```python
from build123d import *

# Parameters (mm, degrees)
SKETCH1_W           = 450
SKETCH1_H           = 25.4
BOSS_EXTRUDE1_DEPTH = 25.4
SKETCH2_W           = 23
SKETCH2_H           = 23
CUT_EXTRUDE1_DEPTH  = 450
CUT_EXTRUDE2_DEPTH  = 25.4


with BuildPart() as part:
    # Sketch1 → Boss-Extrude1 (new body)
    with BuildSketch(Plane(origin=(0, 0, 0), x_dir=(1, 0, 0), z_dir=(0, 1, 0))):
        with Locations((225, 12.7)):
            Rectangle(SKETCH1_W, SKETCH1_H)
    extrude(amount=BOSS_EXTRUDE1_DEPTH)

    # Sketch2 → Cut-Extrude1 (cut)
    with BuildSketch(Plane(origin=(450, 0, 0), x_dir=(0, 0, -1), z_dir=(1, 0, 0))):
        with Locations((12.7, 12.7)):
            Rectangle(SKETCH2_W, SKETCH2_H)
    extrude(amount=-CUT_EXTRUDE1_DEPTH, mode=Mode.SUBTRACT)

    # Sketch3 → Cut-Extrude2 (cut)
    with BuildSketch(Plane(origin=(0, 25.4, 0), x_dir=(1, 0, 0), z_dir=(0, 1, 0))):
        Polygon((0, 0), (25.4, 25.4), (0, 25.4), align=None)
        Polygon((450, 0), (424.6, 25.4), (450, 25.4), align=None)
    extrude(amount=-CUT_EXTRUDE2_DEPTH, mode=Mode.SUBTRACT)


solid = part.part
```
Design review of the part built by this model. Coordinates are the model's own, in mm. A direction names the side the tool comes from. Round coordinates to 2 decimals unless told otherwise and drop trailing zeros. Order: outer loops, then holes, each group sorted by start corner. A loop starts at its lowest first (then second) coordinate and runs counter-clockwise, first axis right, second up. Notation, with made-up numbers: (-18, 62) - (24, 62) arc R28 cw to (24, 83) - close; hole circle Ø9 at (68, 68.5). An arc over 180 degrees is marked (long way). Return JSON: item names as keys, results as strings.
Q1. For pin 1 Ø3 at (x, y) = (88, 7.5) entering from +Z, flat-tipped, find the tip position at first contact; note if it passes through.
Computed values:
{"pin 1": "stops at z = 0"}
Q2. The part is to be moulded in two halves that separate along Z. For faces 3 (the flat face through (222, 13, -25.4)), 4 (the flat face through (222, 13, 0)), 5 (the flat face through (228, 13, -1.2)), 6 (the flat face through (222, 25.4, -13)), say which applies: pulls with the +Z half, pulls with the -Z half, needs draft (parallel to the pull), parting line crosses it, or undercut.
Computed values:
{"face 3": "pulls with the -Z half", "face 4": "pulls with the +Z half", "face 5": "undercut", "face 6": "needs draft"}
Q3. Consider section C-C on x = 411. Write out the cut boundary in (y, z).
Computed values:
{"outline": "(0, -25.4) - (25.4, -25.4) - (25.4, 0) - (0, 0) - close; hole (1.2, -24.2) - (24.2, -24.2) - (24.2, -1.2) - (1.2, -1.2) - close"}
Q4. Machinability: for faces 1 (the flat face through (228, 24.2, -13)), 2 (the flat face through (12, 1, -12)), which of the approach directions +Z, -Z, +X, -X, +Y, -Y give a long, thin tool a straight path to every point of the face, cutting with its end or side? Answer none if there is none.
Computed values:
{"face 1": "+X, -X", "face 2": "-Z, -X, +Y, -Y"}
Q5. Wall thickness on L1, parallel to Z at x = 177, y = 14; L2, parallel to Y at x = 373, z = -17.5; L3, parallel to X at y = 1, z = -11: over which ranges is each line inside the solid? List them lowest first. Write a range as [from, to].
Computed values:
{"L1": "z = [-25.4, -24.2], [-1.2, 0]", "L2": "y = [0, 1.2], [24.2, 25.4]", "L3": "x = [11, 439]"}
Q6. Consider section B-B on y = 15.5. Write out the cut boundary in (x, z), plus the area to 3 significant figures.
Computed values:
{"outline": "(0, 0) - (1.2, -1.2) - (448.8, -1.2) - (450, 0) - close; (24.2, -24.2) - (25.4, -25.4) - (424.6, -25.4) - (425.8, -24.2) - close", "area": "1,020 mm2"}
Q7. Consider section A-A on z = -10. Write out the cut boundary in (x, y).
Computed values:
{"outline": "(10, 0) - (440, 0) - (440, 1.2) - (10, 1.2) - close; (10, 24.2) - (440, 24.2) - (440, 25.4) - (10, 25.4) - close"}
